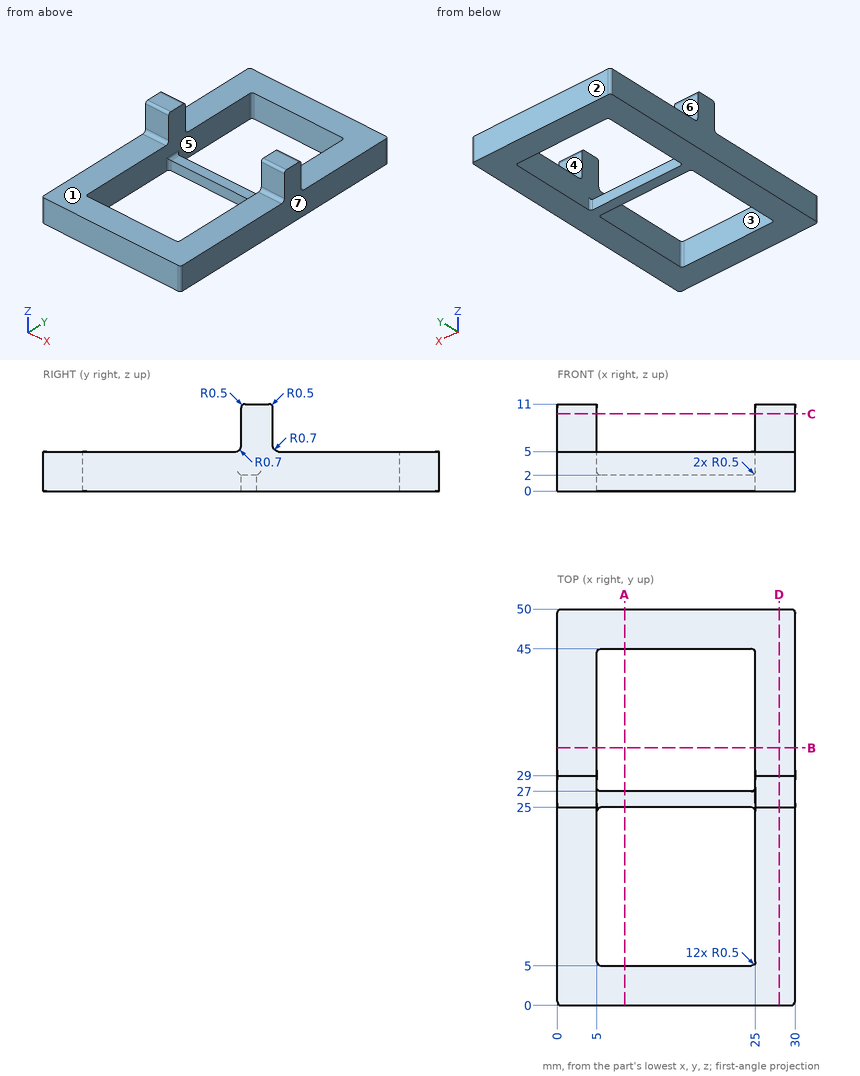
Here's the drawing with two shaded views (mm, measured from the low corner). I have some questions. A direction names the side the tool comes from. Give positions to 0.01 mm unless a question says otherwise; leave off trailing zeros. Loops run counter-clockwise (first coordinate to the right, second up) from the corner with the lowest first, then second, coordinate; pieces in that order, holes last. Notation, with made-up numbers: M -24,88.25 L -3,88.25 A16 ccw -3,108.25 Z; hole C 85,-25.75 d1. An arc over 180 degrees is marked long. One line per item, written item: value. Start each with the question number.
1) I'm going to push flat-ended pins straight in: pin 1 (5 mm diameter, centred on x = 25.5, y = 40, fed in from +Z); pin 2 (1.4 mm diameter, centred on x = 3, z = 8, fed in from -Y); pin 3 (1.4 mm diameter, centred on x = 27.5, z = 7.5, fed in from +Y). Where does each tip first touch, or does it pass through?
2) If we section it at B-B, the plane y = 32.5: Write out the boundary of the cut face in (x, z).
3) If we section it at C-C, the plane z = 9.75: Write out the boundary of the cut face in (x, y), and give its area (3 significant figures).
4) If I drill on line 1 (Y direction, x = 16.25, z = 4.5); line 2 (X direction, y = 32, z = 1.25); line 3 (Y direction, x = 6.75, z = 1), over which ranges is the centre line in solid material (lowest first)? Write a range as [from, to].
5) Thinking about a two-plate mould opening in X: for the marked faces 5, 6 and 7, which applies, +X half, -X half, draft (parallel to the pull), parting line (faces both ways), or undercut?
6) If we section it at D-D, the plane x = 28: Write out the boundary of the cut face in (y, z), and give its area (3 significant figures).
7) On a 3-axis mill with a long thin cutter (end or side, diameter ignored), from which of +Z, -Z, +X, -X, +Y, -Y can I reach the whole of each face in a straight line? I mean the marked faces 1, 2, 3 and 4. Say none if no direction works.
8) If we section it at A-A, the plane x = 8.5: Write out the boundary of the cut face in (y, z).
Completed:
1. pin 1: stops at z = 5
1. pin 2: stops at y = 25
1. pin 3: stops at y = 29
2. outline: M 0,0 L 5,0 L 5,5 L 0,5 Z; M 25,0 L 30,0 L 30,5 L 25,5 Z
3. outline: M 0,25 L 5,25 L 5,29 L 0,29 Z; M 25,25 L 30,25 L 30,29 L 25,29 Z
3. area: 40.0 mm^2
4. line 1: y = [0, 5], [45, 50]
4. line 2: x = [0, 5], [25, 30]
4. line 3: y = [0, 5], [25, 27], [45, 50]
5. face 5: undercut
5. face 6: draft
5. face 7: +X half
6. outline: M 0,0 L 50,0 L 50,5 L 29.7,5 A0.7 cw 29,5.7 L 29,10.5 A0.5 ccw 28.5,11 L 25.5,11 A0.5 ccw 25,10.5 L 25,5.7 A0.7 cw 24.3,5 L 0,5 Z
6. area: 274 mm^2
7. face 1: +Z, +X, -X, -Y
7. face 2: +Z, -Z, +X, -X, +Y
7. face 3: +Z, -Z
7. face 4: +Z, +X, -X, +Y
8. outline: M 0,0 L 5,0 L 5,5 L 0,5 Z; M 25,0 L 27,0 L 27,2 L 25,2 Z; M 45,0 L 50,0 L 50,5 L 45,5 Z
